Geometry check sheet. Reference: the model listing, model coordinates, mm. Face numbers are marked on the shaded views. Coordinates: 2 decimals unless noted, no trailing zeros. Order: outer loops, then holes, each group sorted by start corner. A loop starts at its lowest first (then second) coordinate and runs counter-clockwise, first axis right, second up. Notation, with made-up numbers: (20.25, 81) -> (32.25, 81) arc R20 cw to (32.25, 96) -> close; hole circle Ø8 at (7, -27). An arc over 180 degrees is marked (long way). Answer as CSV lines item,"result". Start each with the question number.
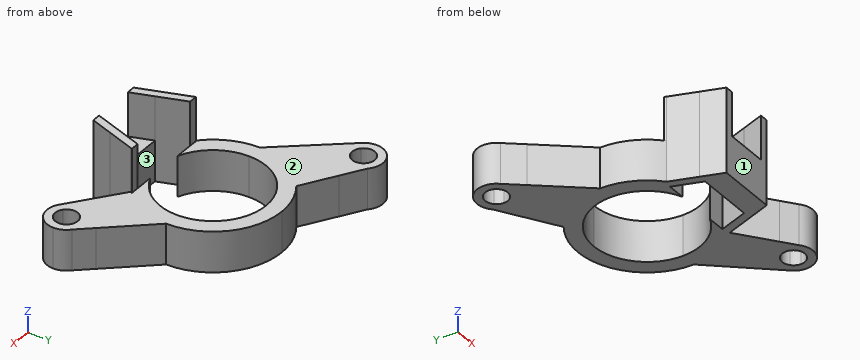
from build123d import *

# Parameters (mm, degrees)
F1_DEPTH = 12
F2_DEPTH = 25
F3_DEPTH = 12


# Not quite as in the source:
# - ends of sketch curves that miss each other by under 0.0002 mm in the source are joined


with BuildPart() as f1:
    # F0 (on Top) → F1 (new body)
    with BuildSketch(Plane.XY):
        with BuildLine():
            ThreePointArc((-53.4150354708, 40.5196217052), (-52.7133447942, 39.4447339634), (-52.4674114416, 38.1848648238))
            Line((-52.4674114416, 38.1848648238), (-50.0674114416, 38.1848649627))
            ThreePointArc((-50.0674114416, 38.1848649627), (-50.4895358529, 40.3473267799), (-51.6939302977, 42.1922833515))
            Line((-51.6939302977, 42.1922833515), (-53.4150354708, 40.5196217052))
        make_face()
        with BuildLine():
            Line((-50.0674114416, 38.1848649627), (-52.4674114416, 38.1848649047))
            ThreePointArc((-52.4674114416, 38.1848649047), (-53.4486037246, 35.8160571069), (-55.8174114415, 34.8348648238))
            Line((-55.8174114415, 34.8348648238), (-55.8174114415, 32.4348648238))
            ThreePointArc((-55.8174114415, 32.4348648238), (-51.7515474497, 34.119000832), (-50.0674114416, 38.1848649627))
        make_face()
        with BuildLine():
            ThreePointArc((-51.6939302977, 42.1922833515), (-50.4895358529, 40.3473267799), (-50.0674114416, 38.1848648238))
            Line((-50.0674114416, 38.1848648238), (-45.2079510631, 38.1848650801))
            Line((-45.2079510631, 38.1848650801), (-51.6939302977, 42.1922833515))
        make_face()
        with BuildLine():
            Line((-45.2079510631, 38.1848650801), (-50.0674114416, 38.1848649627))
            ThreePointArc((-50.0674114416, 38.1848649627), (-51.7515474497, 34.119000832), (-55.8174114415, 32.4348648238))
            Line((-55.8174114415, 32.4348648238), (-55.8174114414, 29.083605512))
            Line((-55.8174114414, 29.083605512), (-44.5532578407, 15.1687110318))
            ThreePointArc((-44.5532578407, 15.1687110318), (-42.1350647352, 24.8048651036), (-35.4555304308, 32.1592477879))
            Line((-35.4555304308, 32.1592477879), (-45.2079510631, 38.1848650801))
        make_face()
        with BuildLine():
            Line((-55.8174114415, 32.4348648238), (-55.8174114415, 34.8348648238))
            ThreePointArc((-55.8174114415, 34.8348648238), (-57.1214560051, 35.0990962362), (-58.2197874124, 35.8501079425))
            Line((-58.2197874124, 35.8501079425), (-59.9408925855, 34.1774462962))
            ThreePointArc((-59.9408925855, 34.1774462962), (-58.0556968865, 32.8883963526), (-55.8174114415, 32.4348648238))
        make_face()
        with BuildLine():
            ThreePointArc((-58.2197874124, 35.8501079425), (-58.1521683229, 40.5872407946), (-53.4150354708, 40.5196217052))
            Line((-53.4150354708, 40.5196217052), (-51.6939302977, 42.1922833515))
            ThreePointArc((-51.6939302977, 42.1922833515), (-59.8248299692, 42.3083459677), (-59.9408925855, 34.1774462962))
            Line((-59.9408925855, 34.1774462962), (-58.2197874124, 35.8501079425))
        make_face()
        with BuildLine():
            Line((-55.8174114414, 29.083605512), (-55.8174114415, 32.4348648238))
            ThreePointArc((-55.8174114415, 32.4348648238), (-58.0556968865, 32.8883963526), (-59.9408925855, 34.1774462962))
            Line((-59.9408925855, 34.1774462962), (-55.8174114414, 29.083605512))
        make_face()
        with BuildLine():
            ThreePointArc((-24.1338443596, 35.5853722206), (-30.0482104313, 34.7100811604), (-35.4555304308, 32.1592477879))
            ThreePointArc((-35.4555304308, 32.1592477879), (-42.1350647352, 24.8048651036), (-44.5532578407, 15.1687110318))
            Line((-44.5532578407, 15.1687110318), (-42.6338443592, 15.1659585535))
            Line((-42.6338443592, 15.1659585535), (-39.8838443592, 15.1659585535))
            ThreePointArc((-39.8838443592, 15.1659585535), (-35.270776163, 26.3028903571), (-24.1338443595, 30.9159585535))
            Line((-24.1338443595, 30.9159585535), (-24.1338443596, 35.5853722206))
        make_face()
        with BuildLine():
            ThreePointArc((-3.7144306922, 15.1659585535), (-9.6951384875, 29.6046644255), (-24.1338443596, 35.5853722206))
            Line((-24.1338443596, 35.5853722206), (-24.1338443595, 30.9159585535))
            ThreePointArc((-24.1338443595, 30.9159585535), (-12.9969125556, 26.3028903573), (-8.3838443592, 15.1659585535))
            Line((-8.3838443592, 15.1659585535), (-5.6338443592, 15.1659585535))
            Line((-5.6338443592, 15.1659585535), (-3.7144306922, 15.1659585535))
        make_face()
        with BuildLine():
            Line((-42.6338443592, 15.1659585535), (-44.5532578407, 15.1687110318))
            ThreePointArc((-44.5532578407, 15.1687110318), (-42.7914410163, 6.8685769492), (-37.807970261, 0.0011725238))
            Line((-37.807970261, 0.0011725238), (-38.0284454354, 0.643162408))
            Line((-38.0284454354, 0.643162408), (-35.5289696075, 0.5919707473))
            Line((-35.5289696075, 0.5919707473), (-42.6338443592, 15.1659585535))
        make_face()
        with BuildLine():
            Line((7.5497227229, 2.079326472), (-3.7144306922, 15.1659585535))
            Line((-3.7144306922, 15.1659585535), (-5.6338443592, 15.1659585535))
            Line((-5.6338443592, 15.1659585535), (-12.7387191109, 0.5919707473))
            Line((-12.7387191109, 0.5919707473), (-10.2387191109, 0.5919707473))
            Line((-10.2387191109, 0.5919707473), (-10.4427343672, 0))
            Line((-10.4427343672, 0), (-0.3331204375, -7.8151351762))
            Line((-0.3331204375, -7.8151351762), (1.9170354556, -7.8151351762))
            ThreePointArc((1.9170354556, -7.8151351762), (3.0939956275, -3.0251503303), (7.549722723, -0.909568585))
            Line((7.549722723, -0.909568585), (7.5497227229, 2.079326472))
        make_face()
        with BuildLine():
            Line((-39.8838443592, 15.1659585535), (-42.6338443592, 15.1659585535))
            Line((-42.6338443592, 15.1659585535), (-35.5289696075, 0.5919707473))
            Line((-35.5289696075, 0.5919707473), (-30.1055593076, 0.5919707473))
            ThreePointArc((-30.1055593076, 0.5919707473), (-37.2127780015, 6.3907665453), (-39.8838443592, 15.1659585535))
        make_face()
        Polygon((-38.0284454354, 0.643162408), (-37.807970261, 0.0011725238), (-35.1236572441, -7.8151351762), (-32.6315665225, -7.8151351762), (-35.5289696075, 0.5919707473), align=None)
        with BuildLine():
            Line((-5.6338443592, 15.1659585535), (-8.3838443592, 15.1659585535))
            ThreePointArc((-8.3838443592, 15.1659585535), (-11.054910717, 6.3907665453), (-18.1621294109, 0.5919707473))
            Line((-18.1621294109, 0.5919707473), (-12.7387191109, 0.5919707473))
            Line((-12.7387191109, 0.5919707473), (-5.6338443592, 15.1659585535))
        make_face()
        with BuildLine():
            Line((11.3813838275, -2.3722765282), (7.5497227229, 2.079326472))
            Line((7.5497227229, 2.079326472), (7.549722723, -0.909568585))
            ThreePointArc((7.549722723, -0.909568585), (9.6004019609, -1.2876774223), (11.3813838275, -2.3722765282))
        make_face()
        Polygon((-32.6315665225, -7.8151351762), (-35.1236572441, -7.8151351762), (-32.8838443592, -14.3371266833), (-30.3838443592, -14.3371266833), align=None)
        Polygon((-10.2387191109, 0.5919707473), (-12.7387191109, 0.5919707473), (-15.636122196, -7.8151351762), (-13.136122196, -7.8151351762), (-10.4427343672, 0), align=None)
        with BuildLine():
            ThreePointArc((11.3813838275, -2.3722765282), (9.6004019609, -1.2876774223), (7.549722723, -0.909568585))
            Line((7.549722723, -0.909568585), (7.549722723, -3.309568585))
            ThreePointArc((7.549722723, -3.309568585), (8.744466279, -3.5298580815), (9.7820818013, -4.1617549519))
            Line((9.7820818013, -4.1617549519), (11.3813838275, -2.3722765282))
        make_face()
        with BuildLine():
            Line((7.549722723, -3.309568585), (7.549722723, -0.909568585))
            ThreePointArc((7.549722723, -0.909568585), (3.0939956275, -3.0251503303), (1.9170354556, -7.8151351762))
            ThreePointArc((1.9170354556, -7.8151351762), (2.5652068364, -9.5261172721), (3.7180616186, -10.9468606418))
            Line((3.7180616186, -10.9468606418), (5.3173636448, -9.1573822181))
            ThreePointArc((5.3173636448, -9.1573822181), (4.4200122196, -5.464825029), (7.549722723, -3.309568585))
        make_face()
        with BuildLine():
            ThreePointArc((13.2997227231, -6.659568585), (12.7982725871, -4.3111171112), (11.3813838275, -2.3722765282))
            Line((11.3813838275, -2.3722765282), (9.7820818013, -4.1617549519))
            ThreePointArc((9.7820818013, -4.1617549519), (10.6075735134, -5.2913403351), (10.8997227231, -6.659568585))
            ThreePointArc((10.8997227231, -6.659568585), (8.917950973, -9.7174193754), (5.3173636448, -9.1573822181))
            Line((5.3173636448, -9.1573822181), (3.7180616186, -10.9468606418))
            ThreePointArc((3.7180616186, -10.9468606418), (9.8981741968, -11.908118449), (13.2997227231, -6.659568585))
        make_face()
        Polygon((-24.1338443592, -7.8151351762), (-32.6315665225, -7.8151351762), (-30.3838443592, -14.3371266833), (-24.1338443592, -14.3371266833), (-24.1338443592, -7.8529477167), align=None)
        Polygon((-13.136122196, -7.8151351762), (-15.636122196, -7.8151351762), (-17.8838443592, -14.3371266833), (-15.3838443592, -14.3371266833), align=None)
        Polygon((-17.8838443592, -14.3371266833), (-15.636122196, -7.8151351762), (-24.1338443592, -7.8151351762), (-24.1338443592, -7.8529477167), (-24.1338443592, -14.3371266833), align=None)
    extrude(amount=F1_DEPTH)

    # F0 (on Top) → F2 (join)
    with BuildSketch(Plane.XY):
        Polygon((-38.0284454354, 0.643162408), (-37.807970261, 0.0011725238), (-35.1236572441, -7.8151351762), (-32.6315665225, -7.8151351762), (-35.5289696075, 0.5919707473), align=None)
        Polygon((-32.6315665225, -7.8151351762), (-35.1236572441, -7.8151351762), (-32.8838443592, -14.3371266833), (-30.3838443592, -14.3371266833), align=None)
        Polygon((-13.136122196, -7.8151351762), (-15.636122196, -7.8151351762), (-17.8838443592, -14.3371266833), (-15.3838443592, -14.3371266833), align=None)
        Polygon((-10.2387191109, 0.5919707473), (-12.7387191109, 0.5919707473), (-15.636122196, -7.8151351762), (-13.136122196, -7.8151351762), (-10.4427343672, 0), align=None)
    extrude(amount=F2_DEPTH)

    # F0 (on Top) → F3 (join)
    with BuildSketch(Plane.XY):
        with BuildLine():
            ThreePointArc((3.7180616186, -10.9468606418), (2.5652068364, -9.5261172721), (1.9170354556, -7.8151351762))
            Line((1.9170354556, -7.8151351762), (-0.3331204375, -7.8151351762))
            Line((-0.3331204375, -7.8151351762), (3.7180616186, -10.9468606418))
        make_face()
    extrude(amount=F3_DEPTH)


solid = f1.part
Q1. Sectioned sample at B-B, the plane y = 18.5. Record the cut outline in (x, z).
Q2. Release check for a two-part mould opening along Y. For the marked faces 1, 2 and 3 record: released by +Y, released by -Y, zero draft, split by the parting line, or undercut.
Q3. Sectioned sample at A-A, the plane z = 15.5. Record the cut outline in (x, y).
Q4. Sectioned sample at C-C, the plane x = -23. Record the cut outline in (y, z), then the cut area to 3 significant figures.
Q5. Go/stop test with flat-tipped pins: pin 1 Ø10 at (y, z) = (29.5, 3) entering from -X; pin 2 Ø2 at (x, y) = (-26, -11) entering from +Z; pin 3 Ø2 at (x, z) = (-11, 6.5) entering from +Y. Record where each tip stops, or that it passes through.
Q6. Thickness scan on L1, parallel to Y at x = -17, z = 11.5; L2, parallel to Z at x = -46, y = 27; L3, parallel to Y at x = -27, z = 2.75. Record the ranges inside material, lowest first.
Q7. Sectioned sample at D-D, the plane z = 8. Record the cut outline in (x, y), then the cut area to 3 significant figures.
Geometry results:
1,outline,"(-47.25, 0) -> (-39.53, 0) -> (-39.53, 12) -> (-47.25, 12) -> close; (-8.74, 0) -> (-3.99, 0) -> (-3.99, 12) -> (-8.74, 12) -> close"
2,face 1,"released by -Y"
2,face 2,"zero draft"
2,face 3,"undercut"
3,outline,"(-38.03, 0.64) -> (-32.88, -14.34) -> (-30.38, -14.34) -> (-35.53, 0.59) -> close; (-17.88, -14.34) -> (-15.38, -14.34) -> (-10.24, 0.59) -> (-12.74, 0.59) -> close"
4,outline,"(-14.34, 0) -> (-7.82, 0) -> (-7.82, 12) -> (-14.34, 12) -> close; (30.88, 0) -> (35.55, 0) -> (35.55, 12) -> (30.88, 12) -> close"
4,area,"134 mm^2"
5,pin 1,"stops at x = -60.23"
5,pin 2,"stops at z = 12"
5,pin 3,"stops at y = 31.59"
6,L1,"y = -14.34 to -7.82, 0.59 to 1.12, 29.21 to 34.3"
6,L2,"z = 0 to 12"
6,L3,"y = -14.34 to -7.82, 30.65 to 35.38"
7,outline,"(-59.94, 34.18) -> (-44.55, 15.17) arc R20.42 ccw to (-37.81, 0) -> (-32.88, -14.34) -> (-15.38, -14.34) -> (-10.44, 0) -> (3.72, -10.95) arc R5.75 ccw to (11.38, -2.37) -> (-3.71, 15.17) arc R20.42 ccw to (-35.46, 32.16) -> (-51.69, 42.19) arc R5.75 ccw to start; hole circle Ø6.7 at (-55.82, 38.18); hole (-35.53, 0.59) -> (-32.63, -7.82) -> (-15.64, -7.82) -> (-12.74, 0.59) -> (-18.16, 0.59) arc R15.75 ccw (long way) to (-30.11, 0.59) -> close; hole circle Ø6.7 at (7.55, -6.66)"
7,area,"1,180 mm^2"
